Source: CAD feature listing. Evaluate the final solid. Frame: model axes, mm. A direction names the side the tool comes from. Coordinates: 2 decimals unless noted, no trailing zeros. Write each loop counter-clockwise with the first axis right and the second up, starting at its lowest first coordinate (ties: lowest second). Pieces come first, ordered by that corner, then holes. Notation, with made-up numbers: (-35.75, 62) - (-22.75, 62) arc R22 ccw to (-22.75, 75) - close; hole circle Ø9 at (32.25, 62.25). An arc over 180 degrees is marked (long way). One line per item, written item: value.
Autodesk Inventor part; units mm, degrees
ref_plane "YZ Plane" through (0, 0, 0) normal (1, 0, 0) x (0, 1, 0)
ref_plane "XZ Plane" through (0, 0, 0) normal (0, 1, 0) x (-1, 0, 0)
ref_plane "XY Plane" through (0, 0, 0) normal (0, 0, 1) x (1, 0, 0)
sketch "Sketch1" plane through (0, 0, 0) normal (0, 1, 0) x (-1, 0, 0)
  circle A0 centre (0, 0) radius 14
  line L0 (-10.2835, 9.5) -> (-15.2835, 9.5)
  line L1 (-15.2835, 9.5) -> (-15.2835, -9.5)
  line L2 (-15.2835, -9.5) -> (-10.2835, -9.5)
  line L3 (-10.2835, -9.5) -> (-10.2835, 9.5)
  point P0 (-10.2835, 0)
  dimension "d0" = 28
  dimension "d3" = 5
  dimension "d4" = 19
extrude "Extrusion1" add sketch "Sketch1" along normal mid plane 19
sketch "Sketch2" plane through (0, 9.5, 0) normal (0, 1, 0) x (1, 0, 0)
  line L0 (0, 0) -> (15.2835, 0) construction
  line L1 (15.2835, -9.5) -> (15.2835, 9.5)
  circle A0 centre (0, 18) radius 2
  arc A1 (10.2835, 9.5) -> (10.2835, -9.5) centre (0, 0) ccw
  line L2 (-3, 13.6748) -> (3, 13.6748)
  line L3 (3, 13.6748) -> (3, 18)
  line L4 (3, 18) -> (-3, 18) construction
  line L5 (-3, 18) -> (-3, 13.6748)
  arc A2 (3, 18) -> (-3, 18) centre (0, 18) ccw
  circle A3 centre (0, -18) radius 2
  line L6 (-3, -13.6748) -> (3, -13.6748)
  line L7 (3, -13.6748) -> (3, -18)
  line L8 (3, -18) -> (-3, -18) construction
  line L9 (-3, -18) -> (-3, -13.6748)
  arc A4 (-3, -18) -> (3, -18) centre (0, -18) ccw
  point P0 (0, 14)
  point P1 (0, 13.6748)
  point P2 (0, -14)
  point P3 (0, -13.6748)
  dimension "d5" = 4
  dimension "d6" = 4
  dimension "d7" = 3
extrude "Extrusion2" add sketch "Sketch2" against normal blind 1 contours A1 L7 A4 L9 | A1 L5 A2 L3
sketch "Sketch3" plane through (0, 9.5, 0) normal (0, 1, 0) x (1, 0, 0)
  circle A0 centre (-8, 0) radius 5
  arc A1 (-3, 13.6748) -> (-3, -13.6748) centre (0, 0) ccw
  point P0 (-14, 0)
  point P1 (-14, 0)
  dimension "d10" = 10
  dimension "d11" = 6
extrude "Extrusion3" add sketch "Sketch3" along normal blind 2
sketch "Sketch4" plane through (-8, 11.5, 0) normal (0, 1, 0) x (1, 0, 0)
  circle A0 centre (0, 0) radius 2.5
  circle A1 centre (0, 0) radius 5
  point P0 (8, 0)
  dimension "d14" = 5
extrude "Extrusion4" add sketch "Sketch4" along normal blind 9 contours A0
sketch "Sketch5" plane through (-8, 20.5, 0) normal (0, 1, 0) x (1, 0, 0)
  circle A0 centre (0, 0) radius 2.5
  circle A1 centre (0, 0) radius 2.5
  line L0 (1.5, -2) -> (1.5, 2)
  line L1 (0, -2.5) -> (0, 2.5) construction
  line L2 (-1.5, -2) -> (-1.5, 2)
  point P0 (8, 0)
  dimension "d19" = 3
extrude "Extrusion5" cut sketch "Sketch5" against normal blind 6 contours A0 L0 | L2 A0
properties part number "smol stepper"
1) Section query D-D on z = 15. Output: boundary loops of the cut face in (x, y), then the cut area to 3 significant figures.
Values found:
outline: (-3, 8.5) - (3, 8.5) - (3, 9.5) - (-3, 9.5) - close
area: 6.00 mm2
2) Draft query along Z for faces 1 (the flat face through (0, 8.5, 15.7)), 2 (the cylindrical face through (-6.66, 14.94, 2.11)), 3 (the cylindrical face through (0, 9, 16)). Return one class per face: released by +Z, released by -Z, zero draft, split by the parting line, or undercut.
Values found:
face 1: zero draft
face 2: split by the parting line
face 3: undercut
3) Reachability of faces 4 (the flat face through (-9.5, 18, 0)), 5 (the flat face through (-3, 9, -16)), 6 (the flat face through (3, 9, 16)), 7 (the flat face through (-6, 11.5, 2)) from +Z, -Z, +X, -X, +Y, -Y: full face, straight path, thin tool, end or side. Return the list, or none.
Values found:
face 4: +Z, -Z, -X, +Y
face 5: -Z, -X, +Y, -Y
face 6: +Z, +X, +Y, -Y
face 7: +Y
4) Contact query for flat-ended pins moving along their axis: P1, Ø14.5, axis at x = -6, z = 9, coming from the +Y side; P2, Ø3, axis at y = 4.5, z = 7.5, coming from the -X side; P3, Ø1.1, axis at y = 9, z = -16.5, coming from the -X side; P4, Ø3, axis at x = -11, y = -4, coming from the +Z side. Output: stop coordinate, or through.
Values found:
P1: y = 20.5
P2: x = -12.65
P3: x = -3
P4: z = 10.28
5) Section query C-C on x = -8. Output: boundary loops of the cut face in (y, z), then the cut area to 3 significant figures.
Values found:
outline: (-9.5, -11.49) - (9.5, -11.49) - (9.5, -5) - (11.5, -5) - (11.5, -2.5) - (20.5, -2.5) - (20.5, 2.5) - (11.5, 2.5) - (11.5, 5) - (9.5, 5) - (9.5, 11.49) - (-9.5, 11.49) - close
area: 502 mm2
6) Material intervals for line 1 (Z direction, x = 0, y = 8.85); line 2 (X direction, y = 9.15, z = 18); line 3 (Y direction, x = -6, z = 5), sorted ascending.
Values found:
line 1: -21 to -20, -16 to 16, 20 to 21
line 2: -3 to -2, 2 to 3
line 3: -9.5 to 9.5
7) Section query B-B on y = 15. Output: boundary loops of the cut face in (x, z).
Values found:
outline: (-9.5, -2) arc R2.5 ccw to (-6.5, -2) - (-6.5, 2) arc R2.5 ccw to (-9.5, 2) - close
8) Section query A-A on x = 0. Output: boundary loops of the cut face in (y, z), then the cut area to 3 significant figures.
Values found:
outline: (-9.5, -14) - (8.5, -14) - (8.5, -16) - (9.5, -16) - (9.5, 16) - (8.5, 16) - (8.5, 14) - (-9.5, 14) - close; (8.5, -21) - (9.5, -21) - (9.5, -20) - (8.5, -20) - close; (8.5, 20) - (9.5, 20) - (9.5, 21) - (8.5, 21) - close
area: 538 mm2
